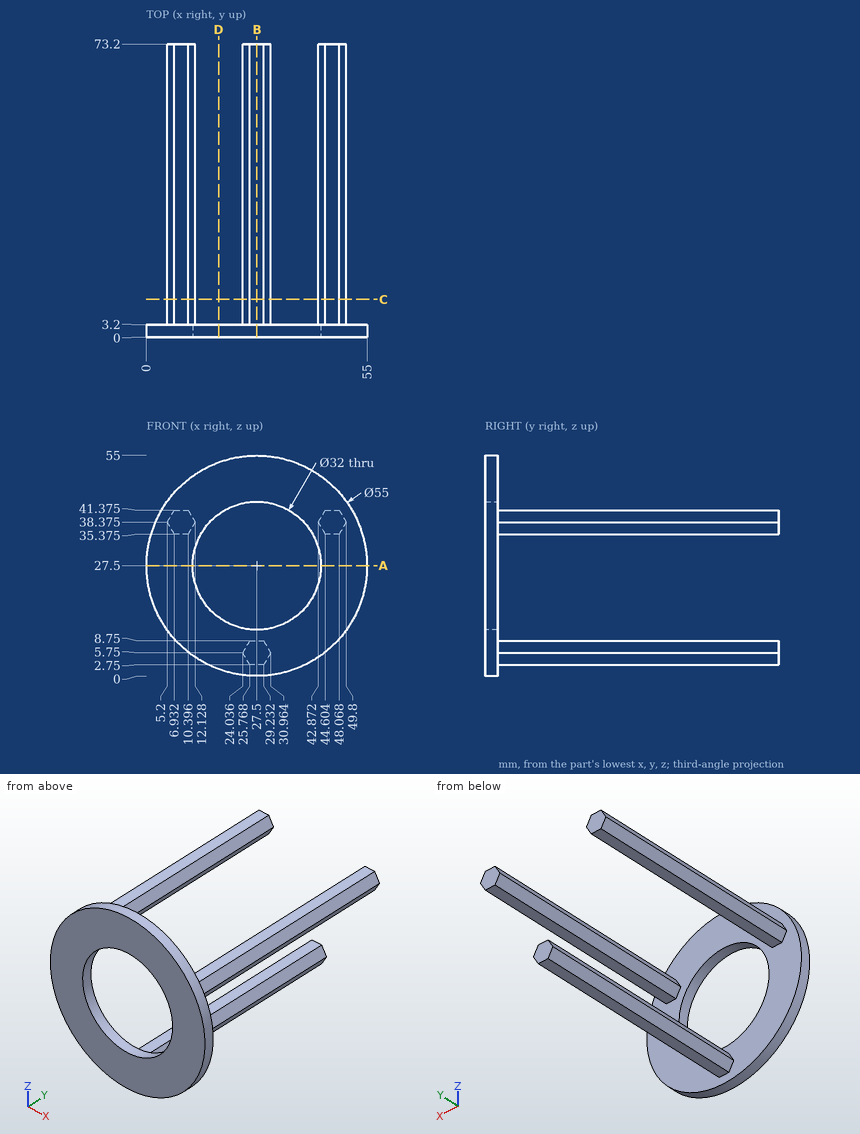
Here's the drawing with two shaded views (mm, measured from the low corner). I have some questions. Give positions to 0.01 mm unless a question says otherwise; leave off trailing zeros. Loops run counter-clockwise (first coordinate to the right, second up) from the corner with the lowest first, then second, coordinate; pieces in that order, holes last. Notation, with made-up numbers: (39, -17) - (59, -17) arc R19 cw to (59, -2) - close; hole circle Ø1 at (16.5, 69). An arc over 180 degrees is marked (long way). Answer in a Markdown table with one row per item. Add a question column.
Q1. Please list where these lines run through material, in increasing order: L1, parallel to X at y = 2.05, z = 27.5; L2, parallel to Y at x = 30.5, z = 10; L3, parallel to X at y = 62.5, z = 7.5. Write a range as from..to.
Q2. If we section it at A-A (z = 27.5): List the corners of the cut face in (x, y) for me, plus the area to 3 significant figures.
Q3. If we section it at D-D (x = 18): List the corners of the cut face in (y, z) for me.
Q4. If we section it at C-C (y = 9.5): List the corners of the cut face in (x, z) for me (3 decimals).
Q5. For pin 1 (4 mm diameter, centred on x = 46, y = 49.5, fed in from +Z) (3 decimals); pin 2 (3 mm diameter, centred on x = 27, y = 37.5, fed in from -Z); pin 3 (4 mm diameter, centred on y = 45.5, z = 43, fed in from +X) (1 decimal), each with a flat end and sliding along its axis, tell me the tip position at first contact or that it passes through.
Q6. If we section it at B-B (x = 27.5): List the corners of the cut face in (y, z) for me, plus the area to 3 significant figures.
The answers:
| question | item | result |
|---|---|---|
| 1 | L1 | x = 0..11.5, 43.5..55 |
| 1 | L2 | y = 0..3.2 |
| 1 | L3 | x = 25.05..29.95 |
| 2 | outline | (0, 0) - (11.5, 0) - (11.5, 3.2) - (0, 3.2) - close; (43.5, 0) - (55, 0) - (55, 3.2) - (43.5, 3.2) - close |
| 2 | area | 73.6 mm^2 |
| 3 | outline | (0, 1.69) - (3.2, 1.69) - (3.2, 14.63) - (0, 14.63) - close; (0, 40.37) - (3.2, 40.37) - (3.2, 53.31) - (0, 53.31) - close |
| 4 | outline | (5.2, 38.375) - (6.932, 35.375) - (10.396, 35.375) - (12.128, 38.375) - (10.396, 41.375) - (6.932, 41.375) - close; (24.036, 5.75) - (25.768, 2.75) - (29.232, 2.75) - (30.964, 5.75) - (29.232, 8.75) - (25.768, 8.75) - close; (42.872, 38.375) - (44.604, 35.375) - (48.068, 35.375) - (49.8, 38.375) - (48.068, 41.375) - (44.604, 41.375) - close |
| 5 | pin 1 | stops at z = 41.375 |
| 5 | pin 2 | stops at z = 2.75 |
| 5 | pin 3 | stops at x = 48.3 |
| 6 | outline | (0, 0) - (3.2, 0) - (3.2, 2.75) - (73.2, 2.75) - (73.2, 8.75) - (3.2, 8.75) - (3.2, 11.5) - (0, 11.5) - close; (0, 43.5) - (3.2, 43.5) - (3.2, 55) - (0, 55) - close |
| 6 | area | 494 mm^2 |
